The model under review builds one solid part; all positions refer to its coordinate system, in mm. A direction names the side the tool comes from. Round coordinates to 2 decimals unless told otherwise and drop trailing zeros. Order: outer loops, then holes, each group sorted by start corner. A loop starts at its lowest first (then second) coordinate and runs counter-clockwise, first axis right, second up.
1) Consider section C-C (y = -3.75). Give the boundary of the cut face in (x, z), then the cut area to 3 significant figures.
2) Consider section B-B (z = -12). Give the boundary of the cut face in (x, y).
3) Mouldability with a two-part tool opening along X and no side actions: class faces 3 (the face through (-21, -6, 2)), 4 (the face through (-10.24, -6.44, -13.36)), 5 (the face through (0, -6, 21)) as pulls with the +X half, pulls with the -X half, needs draft (parallel to the pull), parting line crosses it, or undercut.
4) Consider section A-A (x = 8.7). Give the boundary of the cut face in (y, z).
5) Machinability: for faces 1 (the face through (9, -6, -11)), 2 (the face through (-16, -6, -16)), which of the approach directions +Z, -Z, +X, -X, +Y, -Y give a long, thin tool a straight path to every point of the face, cutting with its end or side? Answer none if there is none.
6) Clearance check with flat-ended pins moving along their axes: P1, Ø6.5, axis at x = -1.3, y = -6.35, coming from the -Z side; P2, Ø2.5, axis at x = -11.1, z = -14.71, coming from the +Y side; P3, Ø1.2, axis at x = 9, y = -6, coming from the -Z side. State where each tip first meets the part, or that it passes through.
7) To check wall thickness, follow L1, parallel to Z at x = 16, y = -11.5; L2, parallel to Y at x = 8.7, z = -14.25; L3, parallel to X at y = -6.35, z = -18.5. State the ranges of each line that lie inside material, in increasing order.
8) Consider section D-D (x = 15). Give the boundary of the cut face in (y, z).
from build123d import *

# Parameters (mm, degrees)
F0_W     = 42
F0_H     = 42
F1_DEPTH = 12.7
F2_R     = 5
F3_SIZE  = 10
F4_R     = 1.6
F5_DEPTH = 25
F6_R     = 2
F7_DEPTH = 10


with BuildPart() as f1:
    # F0 (on Front) → F1 (new body)
    with BuildSketch(Plane.XZ):
        Rectangle(F0_W, F0_H)
    extrude(amount=F1_DEPTH)

    # F2
    f2_edges = [f1.edges().sort_by_distance(p)[0] for p in [
        (21, -6.35, 21),
        (-21, -6.35, 21),
        (21, -6.35, -21),
    ]]
    fillet(f2_edges, radius=F2_R)

    # F3
    f3_edges = [f1.edges().sort_by_distance(p)[0] for p in [
        (-21, -6.35, -21),
    ]]
    chamfer(f3_edges, length=F3_SIZE)

    # F4 (on face) → F5 (cut)
    with BuildSketch(Plane.XZ.offset(12.7)):
        with Locations((-16, 16)):
            Circle(F4_R)
        with Locations((16, -16)):
            Circle(F4_R)
        with Locations((-11.1, -14.710243)):
            Circle(F4_R)
    extrude(amount=-F5_DEPTH, mode=Mode.SUBTRACT)

    # F6 (on face) → F7 (cut)
    with BuildSketch(Plane(origin=(0, 0, -21), x_dir=(1, 0, 0), z_dir=(0, 0, -1))):
        with Locations((8.7, 6.35)):
            Circle(F6_R)
        with Locations((-1.3, 6.35)):
            Circle(F6_R)
    extrude(amount=-F7_DEPTH, mode=Mode.SUBTRACT)


solid = f1.part
Answer below:
1. outline: (-21, -11) - (-11, -21) - (16, -21) arc R5 ccw to (21, -16) - (21, 16) arc R5 ccw to (16, 21) - (-16, 21) arc R5 ccw to (-21, 16) - close; hole circle Ø3.2 at (-16, 16); hole circle Ø3.2 at (-11.1, -14.71); hole circle Ø3.2 at (16, -16)
1. area: 1,670 mm2
2. outline: (-20, -12.7) - (21, -12.7) - (21, 0) - (-20, 0) - close; hole circle Ø4 at (-1.3, -6.35); hole circle Ø4 at (8.7, -6.35)
3. face 3: pulls with the -X half
3. face 4: undercut
3. face 5: needs draft
4. outline: (-12.7, -21) - (-8.35, -21) - (-8.35, -11) - (-4.35, -11) - (-4.35, -21) - (0, -21) - (0, 21) - (-12.7, 21) - close
5. face 1: -Z
5. face 2: -Z, -X, +Y, -Y
6. P1: stops at z = -21
6. P2: passes through
6. P3: stops at z = -11
7. L1: z = -21 to -17.6, -14.4 to 21
7. L2: y = -12.7 to -8.35, -4.35 to 0
7. L3: x = -13.5 to -3.3, 0.7 to 6.7, 10.7 to 20.33
8. outline: (-12.7, -21) - (0, -21) - (0, -17.25) - (-12.7, -17.25) - close; (-12.7, -14.75) - (0, -14.75) - (0, 21) - (-12.7, 21) - close
